The model under review builds one solid part; all positions refer to its coordinate system, in mm. A direction names the side the tool comes from. Round coordinates to 2 decimals unless told otherwise and drop trailing zeros. Write each loop counter-clockwise with the first axis right and the second up, starting at its lowest first coordinate (ties: lowest second). Pieces come first, ordered by that corner, then holes.
Item 1: Add section D-D (x = -3). Give the boundary of the cut face in (y, z), plus the area to 3 significant figures.
Item 2: To check wall thickness, follow L1, parallel to X at y = 0.5, z = 0; L2, parallel to X at y = -1.25, z = 0; L3, parallel to X at y = 0.25, z = -5.5. State the ranges of each line that lie inside material, in increasing order.
Item 3: Draft analysis for pull direction Z (two halves, no side actions). For faces 1 (the face through (0, -5, 7.5)), 2 (the face through (7.56, -2.61, 0.54)), 3 (the face through (-23.12, 2.46, -13.75)), 4 (the face through (16.99, 2.46, -14.54)), state which applies: +Z half, -Z half, draft (parallel to the pull), parting line (faces both ways), or undercut.
Item 4: Add section A-A (x = -20.5). Give the boundary of the cut face in (y, z), plus the area to 3 significant figures.
Item 5: Add section B-B (z = 0). Give the boundary of the cut face in (x, y), plus the area to 3 significant figures.
Item 6: Clearance check with flat-ended pins moving along their axes: pin 1 Ø1.5 at (x, y) = (-12.5, -6) entering from +Z; pin 2 Ø3 at (x, y) = (2.5, -3) entering from +Z. State where each tip first meets the part, or that it passes through.
Item 7: Add section C-C (y = -4.75). Give the boundary of the cut face in (x, z).
Item 8: Machinability: for faces 5 (the face through (0, -5, -7.5)), 6 (the face through (17.5, -4.93, 0.16)), 7 (the face through (-26.952, 2, 0)), which of the approach directions +Z, -Z, +X, -X, +Y, -Y give a long, thin tool a straight path to every point of the face, cutting with its end or side? Answer none if there is none.
```python
from build123d import *

# Parameters (mm, degrees)
BOSS_EXTRUDE1_DEPTH = 5
BOSS_EXTRUDE2_DEPTH = 10
SKETCH3_R           = 2.5
CUT_EXTRUDE1_DEPTH  = 16


with BuildPart() as part:
    # Sketch1 → Boss-Extrude1 (new body)
    # profile 1 of 2: a face of its own
    with BuildSketch(Plane(origin=(0, 0, 0), x_dir=(1, 0, 0), z_dir=(0, 1, 0))):
        with BuildLine():
            ThreePointArc((10, 17.391059627), (17.071067812, 14.462127439), (20, 7.391059627))
            Line((20, 7.391059627), (20, -7.391059627))
            ThreePointArc((20, -7.391059627), (17.071067812, -14.462127439), (10, -17.391059627))
            Line((10, -17.391059627), (-22.161548626, -17.391059627))
            ThreePointArc((-22.161548626, -17.391059627), (-29.232616438, -14.462127439), (-32.161548626, -7.391059627))
            Line((-32.161548626, -7.391059627), (-32.161548626, 7.391059627))
            ThreePointArc((-32.161548626, 7.391059627), (-29.232616438, 14.462127439), (-22.161548626, 17.391059627))
            Line((-22.161548626, 17.391059627), (10, 17.391059627))
        make_face()
        with BuildLine():
            ThreePointArc((-26.951571496, -10), (-23.201571496, -13.75), (-19.451571496, -10))
            Line((-19.451571496, -10), (-19.451571496, 10))
            ThreePointArc((-19.451571496, 10), (-23.201571496, 13.75), (-26.951571496, 10))
            Line((-26.951571496, 10), (-26.951571496, -10))
        make_face(mode=Mode.SUBTRACT)
        with BuildLine():
            ThreePointArc((10, -7.5), (17.5, 0), (10, 7.5))
            Line((10, 7.5), (-10, 7.5))
            ThreePointArc((-10, 7.5), (-17.5, 0), (-10, -7.5))
            Line((-10, -7.5), (10, -7.5))
        make_face(mode=Mode.SUBTRACT)
    # profile 2 of 2: a face of its own
    with BuildSketch(Plane(origin=(0, 0, 0), x_dir=(1, 0, 0), z_dir=(0, 1, 0))):
        with BuildLine():
            Line((-10, -7.5), (10, -7.5))
            ThreePointArc((10, -7.5), (17.5, 0), (10, 7.5))
            Line((10, 7.5), (-10, 7.5))
            ThreePointArc((-10, 7.5), (-17.5, 0), (-10, -7.5))
        make_face()
    extrude(amount=BOSS_EXTRUDE1_DEPTH)

    # Sketch1_3 → Boss-Extrude2 (add)
    with BuildSketch(Plane(origin=(0, 0, 0), x_dir=(1, 0, 0), z_dir=(0, 1, 0))):
        with BuildLine():
            Line((-10, -7.5), (10, -7.5))
            ThreePointArc((10, -7.5), (17.5, 0), (10, 7.5))
            Line((10, 7.5), (-10, 7.5))
            ThreePointArc((-10, 7.5), (-17.5, 0), (-10, -7.5))
        make_face()
    extrude(amount=-BOSS_EXTRUDE2_DEPTH)

    # Sketch3 → Cut-Extrude1 (cut)
    with BuildSketch(Plane.XZ.offset(10)):
        with Locations(Location((10, 0, 0), (0, 0, 270))):
            Circle(SKETCH3_R)
    extrude(amount=-CUT_EXTRUDE1_DEPTH, mode=Mode.SUBTRACT)


solid = part.part
```
Numbers:
1. outline: (-10, -7.5) - (0, -7.5) - (0, -17.39) - (5, -17.39) - (5, 17.39) - (0, 17.39) - (0, 7.5) - (-10, 7.5) - close
1. area: 324 mm2
2. L1: x = -32.16 to -26.95, -19.45 to 7.5, 12.5 to 20
2. L2: x = -17.5 to 7.5, 12.5 to 17.5
2. L3: x = -32.16 to -26.95, -19.45 to 20
3. face 1: +Z half
3. face 2: undercut
3. face 3: undercut
3. face 4: -Z half
4. outline: (0, -17.39) - (5, -17.39) - (5, -12.6) - (0, -12.6) - close; (0, 12.6) - (5, 12.6) - (5, 17.39) - (0, 17.39) - close
4. area: 47.9 mm2
5. outline: (-32.16, 0) - (-26.95, 0) - (-26.95, 5) - (-32.16, 5) - close; (-19.45, 0) - (-17.5, 0) - (-17.5, -10) - (7.5, -10) - (7.5, 5) - (-19.45, 5) - close; (12.5, -10) - (17.5, -10) - (17.5, 0) - (20, 0) - (20, 5) - (12.5, 5) - close
5. area: 498 mm2
6. pin 1: stops at z = 7.29
6. pin 2: stops at z = 7.5
7. outline: (-10, -7.5) - (10, -7.5) arc R7.5 ccw to (10, 7.5) - (-10, 7.5) arc R7.5 ccw to start; hole circle Ø5 at (10, 0)
8. face 5: -Z, +X, -X, -Y
8. face 6: +X, -Y
8. face 7: +Y, -Y
